CAD build for the part. Positions are in the model's coordinates, mm. A direction names the side the tool comes from. Round coordinates to 2 decimals unless told otherwise and drop trailing zeros. Loops run counter-clockwise (first coordinate to the right, second up) from the corner with the lowest first, then second, coordinate; pieces in that order, holes last. Notation, with made-up numbers: (-6.75, 70.5) - (37.25, 70.5) arc R19 ccw to (37.25, 105.5) - close; hole circle Ø11 at (4, -4). An arc over 180 degrees is marked (long way). Use one line per item in the form item = value.
from build123d import *

# Parameters (mm, degrees)
F0_R     = 7.75
F0_R_2   = 5.75
F1_DEPTH = 20
F2_R     = 12.5
F2_R_2   = 7.75
F3_DEPTH = 3
F4_SIZE  = 1.99999


# Not quite as in the source:
# - a fillet or chamfer is up to 0.001 mm smaller than in the source, because OpenCascade refuses the exact size


with BuildPart() as f1:
    # F0 (on Top) → F1 (new body)
    with BuildSketch(Plane.XY):
        Circle(F0_R)
        Circle(F0_R_2, mode=Mode.SUBTRACT)
    extrude(amount=F1_DEPTH)

    # F2 (on Top) → F3 (join)
    with BuildSketch(Plane.XY):
        Circle(F2_R)
        Circle(F2_R_2, mode=Mode.SUBTRACT)
    extrude(amount=F3_DEPTH)

    # F4 (size 2 in the source; OpenCascade refuses exactly that, so slightly less here)
    f4_edges = [f1.edges().sort_by_distance(p)[0] for p in [
        (-7.75, 0, 20),
    ]]
    chamfer(f4_edges, length=F4_SIZE)


solid = f1.part
1) Flat gauge pins, fed straight in: pin 1 (5 mm diameter, centred on y = 2, z = 8, fed in from +X); pin 2 (7 mm diameter, centred on x = 0, y = 0, fed in from -Z) (3 decimals); pin 3 (3 mm diameter, centred on y = 4.5, z = 6, fed in from -X). Where does each tip first touch, or does it go through?
Report:
pin_1 = 7.75
pin_2 = through
pin_3 = -7.15
2) Drill centre lines: probe 1 along Y at (x, z) = (0, 6.25); probe 2 along Z at (x, y) = (3.75, -10); probe 3 along X at (y, z) = (5.25, 16). Where is each one in solid material? Low to high.
Report:
probe_1 = -7.75 to -5.75, 5.75 to 7.75
probe_2 = 0 to 3
probe_3 = -5.7 to -2.35, 2.35 to 5.7
3) Slice it at D-D (y = 9.25). Write the cut outline in (x, z), plus the area to 3 significant figures.
Report:
outline = (-8.41, 0) - (8.41, 0) - (8.41, 3) - (-8.41, 3) - close
area = 50.4 mm^2
4) Two-plate mould, pull along Y, no slides. Class faces 1 (the cylindrical face through (-0.75, 5.7, 9.86)), 2 (the cylindrical face through (-1.009, 7.684, 10.395)), 3 (the flat face through (2.6, -5.4, 0)): +Y half, -Y half, draft (parallel to the pull), parting line (faces both ways), or undercut.
Report:
face_1 = undercut
face_2 = parting line
face_3 = draft
5) Tool access for faces 4 (the flat face through (0, -8, 3)), 5 (the cylindrical face through (11.923, 3.755, 1.479)): list every direction of +Z, -Z, +X, -X, +Y, -Y with a clear straight run to the whole face (end or side of a thin tool).
Report:
face_4 = +Z
face_5 = +Z, -Z
6) Slice it at C-C (z = 11). Write the cut outline in (x, y).
Report:
outline = circle Ø15.5 at (0, 0); hole circle Ø11.5 at (0, 0)
